```python
from build123d import *

# Parameters (mm, degrees)
F1_DEPTH    = 6
F2_DEPTH    = 11.5
F3_SIZE     = 4
F4_W        = 6
F4_H        = 45
F5_DEPTH    = 25
F6_SIZE     = 5.99999
F8_START    = -6
F7_W        = 2
F7_H        = 3
F8_DEPTH    = 7
F9_R        = 1
F10_R       = 1
F11_R       = 2
F12_SIZE2   = 2
F12_SIZE    = 5
F12_2_SIZE2 = 2
F12_2_SIZE  = 5
F13_W       = 3
F13_H       = 7
F14_DEPTH   = 4


# Not quite as in the source:
# - a fillet or chamfer is up to 0.001 mm smaller than in the source, because OpenCascade refuses the exact size


with BuildPart() as f1:
    # F0 (on Front) → F1 (new body)
    with BuildSketch(Plane.XZ):
        with BuildLine():
            Line((-4, 36.76), (-20, 36.76))
            Line((-20, 36.76), (-20, -36.76))
            Line((-20, -36.76), (-4, -36.76))
            Line((-4, -36.76), (-4, -31))
            ThreePointArc((-4, -31), (-5, -28), (-4, -25))
            Line((-4, -25), (-4, -3))
            ThreePointArc((-4, -3), (-5, 0), (-4, 3))
            Line((-4, 3), (-4, 25))
            ThreePointArc((-4, 25), (-5, 28), (-4, 31))
            Line((-4, 31), (-4, 36.76))
        make_face()
        with BuildLine():
            Line((20, 36.76), (-4, 36.76))
            Line((-4, 36.76), (-4, 31))
            ThreePointArc((-4, 31), (1.5811388301, 32.7434164903), (5, 28))
            ThreePointArc((5, 28), (1.5811388301, 23.2565835097), (-4, 25))
            Line((-4, 25), (-4, 3))
            ThreePointArc((-4, 3), (1.5811388301, 4.7434164903), (5, 0))
            ThreePointArc((5, 0), (1.5811388301, -4.7434164903), (-4, -3))
            Line((-4, -3), (-4, -25))
            ThreePointArc((-4, -25), (1.5811388301, -23.2565835097), (5, -28))
            ThreePointArc((5, -28), (1.5811388301, -32.7434164903), (-4, -31))
            Line((-4, -31), (-4, -36.76))
            Line((-4, -36.76), (20, -36.76))
            Line((20, -36.76), (20, 36.76))
        make_face()
        with BuildLine():
            Line((-4, 25), (-4, 31))
            ThreePointArc((-4, 31), (-5, 28), (-4, 25))
        make_face()
        with BuildLine():
            Line((-4, -3), (-4, 3))
            ThreePointArc((-4, 3), (-5, 0), (-4, -3))
        make_face()
        with BuildLine():
            ThreePointArc((-4, -25), (-5, -28), (-4, -31))
            Line((-4, -31), (-4, -25))
        make_face()
    extrude(amount=F1_DEPTH)

    # F0 (on Front) → F2 (join)
    with BuildSketch(Plane.XZ):
        with BuildLine():
            Line((20, 36.76), (-4, 36.76))
            Line((-4, 36.76), (-4, 31))
            ThreePointArc((-4, 31), (1.5811388301, 32.7434164903), (5, 28))
            ThreePointArc((5, 28), (1.5811388301, 23.2565835097), (-4, 25))
            Line((-4, 25), (-4, 3))
            ThreePointArc((-4, 3), (1.5811388301, 4.7434164903), (5, 0))
            ThreePointArc((5, 0), (1.5811388301, -4.7434164903), (-4, -3))
            Line((-4, -3), (-4, -25))
            ThreePointArc((-4, -25), (1.5811388301, -23.2565835097), (5, -28))
            ThreePointArc((5, -28), (1.5811388301, -32.7434164903), (-4, -31))
            Line((-4, -31), (-4, -36.76))
            Line((-4, -36.76), (20, -36.76))
            Line((20, -36.76), (20, 36.76))
        make_face()
        with BuildLine():
            Line((-4, 36.76), (-20, 36.76))
            Line((-20, 36.76), (-20, -36.76))
            Line((-20, -36.76), (-4, -36.76))
            Line((-4, -36.76), (-4, -31))
            ThreePointArc((-4, -31), (-5, -28), (-4, -25))
            Line((-4, -25), (-4, -3))
            ThreePointArc((-4, -3), (-5, 0), (-4, 3))
            Line((-4, 3), (-4, 25))
            ThreePointArc((-4, 25), (-5, 28), (-4, 31))
            Line((-4, 31), (-4, 36.76))
        make_face()
    extrude(amount=-F2_DEPTH)

    # F3
    f3_edges = [f1.edges().sort_by_distance(p)[0] for p in [
        (20, 2.75, -36.76),
        (-20, 2.75, -36.76),
    ]]
    chamfer(f3_edges, length=F3_SIZE)

    # F4 (on Front) → F5 (cut, symmetric)
    with BuildSketch(Plane.XZ):
        with Locations((-17, 1.1105760932)):
            Rectangle(F4_W, F4_H)
    extrude(amount=F5_DEPTH, both=True, mode=Mode.SUBTRACT)

    # F6 (size 6 in the source; OpenCascade refuses exactly that, so slightly less here)
    f6_edges = [f1.edges().sort_by_distance(p)[0] for p in [
        (-20, 2.75, 23.610576),
        (-20, 2.75, -21.389424),
    ]]
    chamfer(f6_edges, length=F6_SIZE)

    # F7 (on Right) → F8 (join)
    with BuildSketch(Plane.YZ.offset(F8_START)):
        with Locations((-7, 33)):
            Rectangle(F7_W, F7_H)
        with Locations((-7, 23)):
            Rectangle(F7_W, F7_H)
        with Locations((-7, 5)):
            Rectangle(F7_W, F7_H)
        with Locations((-7, -5)):
            Rectangle(F7_W, F7_H)
        with Locations((-7, -23)):
            Rectangle(F7_W, F7_H)
        with Locations((-7, -33)):
            Rectangle(F7_W, F7_H)
    extrude(amount=-F8_DEPTH)

    # F9
    f9_edges = [f1.edges().sort_by_distance(p)[0] for p in [
        (-13, -7, -34.5),
    ]]
    fillet(f9_edges, radius=F9_R)

    # F10
    f10_edges = [f1.edges().sort_by_distance(p)[0] for p in [
        (-6, -7, -34.5),
        (-13, -7, -31.5),
        (-6, -7, -31.5),
        (-9.5, -8, -31.5),
        (-9, -8, -34.5),
        (-6, -8, -33),
        (-6, -7, -24.5),
        (-13, -7, -24.5),
        (-13, -7, -21.5),
        (-6, -7, -21.5),
        (-9.5, -8, -21.5),
        (-9.5, -8, -24.5),
        (-6, -8, -23),
        (-13, -8, -23),
        (-6, -7, -6.5),
        (-13, -7, -6.5),
        (-13, -7, -3.5),
        (-6, -7, -3.5),
        (-9.5, -8, -6.5),
        (-9.5, -8, -3.5),
        (-6, -8, -5),
        (-13, -8, -5),
        (-13, -7, 3.5),
        (-6, -7, 3.5),
        (-6, -7, 6.5),
        (-13, -7, 6.5),
        (-9.5, -8, 6.5),
        (-9.5, -8, 3.5),
        (-13, -8, 5),
        (-6, -8, 5),
        (-13, -7, 21.5),
        (-6, -7, 21.5),
        (-6, -7, 24.5),
        (-13, -7, 24.5),
        (-9.5, -8, 24.5),
        (-9.5, -8, 21.5),
        (-6, -8, 23),
        (-13, -8, 23),
        (-9.5, -8, 31.5),
        (-13, -7, 31.5),
        (-6, -7, 31.5),
        (-6, -8, 33),
        (-13, -8, 33),
        (-9.5, -8, 34.5),
        (-13, -7, 34.5),
        (-6, -7, 34.5),
    ]]
    fillet(f10_edges, radius=F10_R)

    # F11
    f11_edges = [f1.edges().sort_by_distance(p)[0] for p in [
        (-20, 2.75, 36.76),
        (20, 2.75, 36.76),
    ]]
    fillet(f11_edges, radius=F11_R)

    # F12
    f12_edges = [f1.edges().sort_by_distance(p)[0] for p in [
        (20, -6, 1),
    ]]
    f12_side = f1.faces().sort_by_distance((20, 2.75, 1))[0]
    chamfer(f12_edges, length=F12_SIZE, length2=F12_SIZE2, reference=f12_side)

    # F12#2
    f12_2_edges = [f1.edges().sort_by_distance(p)[0] for p in [
        (0, -6, -36.76),
    ]]
    f12_2_side = f1.faces().sort_by_distance((0, 2.75, -36.76))[0]
    chamfer(f12_2_edges, length=F12_2_SIZE, length2=F12_2_SIZE2, reference=f12_2_side)

    # F13 (on face) → F14 (cut)
    with BuildSketch(Plane(origin=(-14, 0, 0), x_dir=(0, -1, 0), z_dir=(-1, 0, 0))):
        with Locations((-8, 12.6105760932)):
            Rectangle(F13_W, F13_H)
        with Locations((-8, -10.3894239068)):
            Rectangle(F13_W, F13_H)
    extrude(amount=-F14_DEPTH, mode=Mode.SUBTRACT)


solid = f1.part
```
The listing builds one solid part. Answer for the finished solid, in the listing's coordinates (mm). A direction names the side the tool comes from. Coordinates: 2 decimals unless noted, no trailing zeros. Loops run counter-clockwise (first coordinate to the right, second up) from the corner with the lowest first, then second, coordinate; pieces in that order, holes last. Notation, with made-up numbers: (-32.5, 72.25) - (-16.5, 72.25) arc R8 ccw to (-16.5, 77.25) - close; hole circle Ø6 at (58, 6.25). An arc over 180 degrees is marked (long way). Write item = value, one per line.
1) Determine the mould class of faces 4 (the face through (17.97, 4.57, -34.79)), 5 (the face through (5, 3, 0)), 6 (the face through (-14, 3, 1)) for opening direction X: pulls with the +X half, pulls with the -X half, needs draft (parallel to the pull), parting line crosses it, or undercut.
Responses:
face_4 = pulls with the +X half
face_5 = undercut
face_6 = pulls with the -X half
2) Which of the six approach directions +Z, -Z, +X, -X, +Y, -Y give full straight-line access (tool end or side, diameter ignored) to faces 1 (the face through (-17.04, 2.63, 26.65)), 2 (the face through (-4, -3, 28)), 3 (the face through (-10, 8, -10))?
Responses:
face_1 = -X, +Y, -Y
face_2 = +Y, -Y
face_3 = -X
3) Each of these flat-tipped pins is pushed along its axis until it touches: P1, Ø0.8, axis at x = -4.5, z = -28.5, coming from the +Y side; P2, Ø0.5, axis at x = -10, y = -6.5, coming from the +Z side; P3, Ø6, axis at y = -4.5, z = -15, coming from the -X side. Where does it stop, or does it pass through?
Responses:
P1 = 0
P2 = 34.5
P3 = -14
4) Section C-C (x = -15) is taken. Determine the outline of the cut face in (y, z).
Responses:
outline = (-6, -34.76) - (-1, -36.76) - (11.5, -36.76) - (11.5, -22.39) - (-6, -22.39) - close; (-6, 24.61) - (11.5, 24.61) - (11.5, 36.76) - (-1, 36.76) - (-6, 34.76) - close
5) Section B-B (y = 8) is taken. Count the separate pieces of the cut face and the enclosed holes in it, plus the area to 3 significant figures.
Responses:
separate_pieces = 1
enclosed_holes = 3
area = 2,330 mm^2
6) Section D-D (z = 11.5) is taken. Determine the outline of the cut face in (x, y), plus the area to 3 significant figures.
Responses:
outline = (-14, -6) - (18, -6) - (20, -1) - (20, 11.5) - (-14, 11.5) - (-14, 9.5) - (-10, 9.5) - (-10, 6.5) - (-14, 6.5) - close
area = 578 mm^2
7) Find the intervals of material crossed by line 1 along Z through (x, y) = (0, 6.75); line 2 along X through (y, z) = (2.5, -28); line 3 along Z through (x, y) = (2.5, -0.25), in increasing order.
Responses:
line_1 = -36.76 to -33, -23 to -5, 5 to 23, 33 to 36.76
line_2 = -20 to -5, 5 to 20
line_3 = -36.76 to -32.33, -23.67 to -4.33, 4.33 to 23.67, 32.33 to 36.76
8) Section A-A (z = 0) is taken. Determine the outline of the cut face in (x, y), plus the area to 3 significant figures.
Responses:
outline = (-14, -6) - (-4, -6) - (-4, 0) - (-5, 0) - (-5, 11.5) - (-14, 11.5) - close; (5, -6) - (18, -6) - (20, -1) - (20, 11.5) - (5, 11.5) - close
area = 421 mm^2
